```python
from build123d import *

# Parameters (mm, degrees)
ESBO_O1_R                = 17.5
ESBO_O1_R_2              = 10
RESSALTO_EXTRUS_O1_DEPTH = 9.525
CHANFRO1_SIZE            = 1


with BuildPart() as part:
    # Esboço1 → Ressalto-extrusão1 (new body)
    with BuildSketch(Plane.XY):
        Circle(ESBO_O1_R)
        Circle(ESBO_O1_R_2, mode=Mode.SUBTRACT)
    extrude(amount=RESSALTO_EXTRUS_O1_DEPTH)

    # Chanfro1
    chanfro1_edges = [part.edges().sort_by_distance(p)[0] for p in [
        (-17.5, 0, 0),
        (-17.5, 0, 9.525),
        (-10, 0, 0),
        (-10, 0, 9.525),
    ]]
    chamfer(chanfro1_edges, length=CHANFRO1_SIZE)


solid = part.part
```
Verification items for the finished model (mm, model axes). Give positions to 0.01 mm unless a question says otherwise; leave off trailing zeros. Order: outer loops, then holes, each group sorted by start corner. A loop starts at its lowest first (then second) coordinate and runs counter-clockwise, first axis right, second up. Notation, with made-up numbers: (1, 89.25) - (34, 89.25) arc R20 ccw to (34, 96.25) - close; hole circle Ø8 at (50, 66.25). An arc over 180 degrees is marked (long way). Answer as CSV lines item,"result". Start each with the question number.
Item 1: Section check C-C, the plane z = 6.5. Record the boundary of the cut face in (x, y).
Item 2: Gauge pin test, flat end, axial feed: pin 1 (4 mm diameter, centred on y = 13.5, z = 4, fed in from +X). Record the tip position at first contact, or that the pin passes through.
Item 3: Section check A-A, the plane x = 0. Record the boundary of the cut face in (y, z) (3 decimals), plus the area to 3 significant figures.
Item 4: Material ranges on L1, parallel to Y at x = 0, z = 4.5; L2, parallel to Y at x = -2, z = 2, recorded low to high.
Item 5: Mould release check, pull along Y, two halves, no side actions. Record for faces 1 (the face through (-13.887, -10.648, 4.71)), 2 (the face through (-2.17, -9.76, 4.71)), 3 (the face through (3, -11, 9.525)): released by +Y, released by -Y, zero draft, split by the parting line, or undercut.
Filled in:
1,outline,"circle Ø35 at (0, 0); hole circle Ø20 at (0, 0)"
2,pin 1,"x = 13.19"
3,outline,"(-17.5, 1) - (-16.5, 0) - (-11, 0) - (-10, 1) - (-10, 8.525) - (-11, 9.525) - (-16.5, 9.525) - (-17.5, 8.525) - close; (10, 1) - (11, 0) - (16.5, 0) - (17.5, 1) - (17.5, 8.525) - (16.5, 9.525) - (11, 9.525) - (10, 8.525) - close"
3,area,"139 mm^2"
4,L1,"-17.5 to -10, 10 to 17.5"
4,L2,"-17.39 to -9.8, 9.8 to 17.39"
5,face 1,"split by the parting line"
5,face 2,"undercut"
5,face 3,"zero draft"
